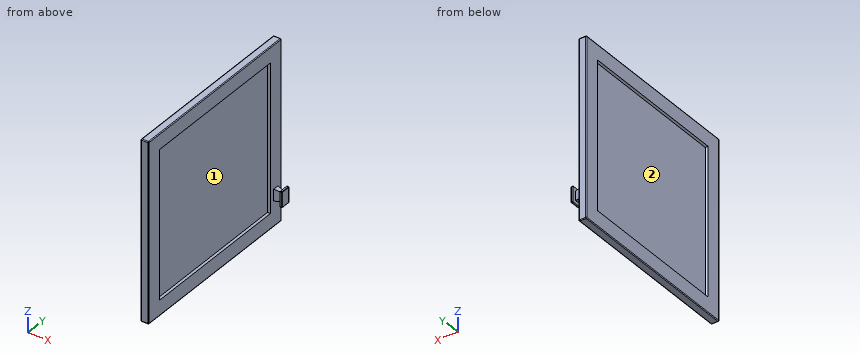
```python
from build123d import *

# Parameters (mm, degrees)
SKETCH1_W               = 479
SKETCH1_H               = 460
BOSS_EXTRUDE1_DEPTH     = 10
SKETCH2_W               = 399
SKETCH2_H               = 380
CUT_EXTRUDE1_DEPTH      = 5
CUT_EXTRUDE1_DRAFT      = -30
MIRROR1_COPY_1_SKETCH_W = 399
MIRROR1_COPY_1_SKETCH_H = 380
MIRROR1_COPY_1_DEPTH    = 5
MIRROR1_COPY_1_DRAFT    = -30
SKETCH3_W               = 15
SKETCH3_H               = 30
BOSS_EXTRUDE2_DEPTH     = 20
BOSS_EXTRUDE2_TAPER     = 10
SKETCH4_W               = 25
SKETCH4_H               = 40
BOSS_EXTRUDE3_DEPTH     = 5
FILLET3_R               = 2
FILLET4_R               = 1


with BuildPart() as part:
    # Sketch1 → Boss-Extrude1 (new, symmetric)
    with BuildSketch(Plane.YZ):
        with Locations((239.5, 230)):
            Rectangle(SKETCH1_W, SKETCH1_H)
    extrude(amount=BOSS_EXTRUDE1_DEPTH, both=True)


with BuildPart() as cut_extrude1_tool:
    # Sketch2 → Cut-Extrude1 (with draft: the straight prism first)
    with BuildSketch(Plane.YZ.offset(10)):
        with Locations((239.5, 230)):
            Rectangle(SKETCH2_W, SKETCH2_H)
    extrude(amount=-CUT_EXTRUDE1_DEPTH)
    # Cut-Extrude1: the draft: its side faces are tilted about the plane it starts from
    cut_extrude1_sides = [cut_extrude1_tool.faces().sort_by_distance(p)[0] for p in [
        (7.5, 40, 230),
        (7.5, 239.5, 40),
        (7.5, 439, 230),
        (7.5, 239.5, 420),
    ]]
    draft(cut_extrude1_sides, Plane.YZ.offset(10), CUT_EXTRUDE1_DRAFT)


with BuildPart() as part_1:
    add(part.part)

    # Cut-Extrude1: cut by cut_extrude1_tool
    add(cut_extrude1_tool.part, mode=Mode.SUBTRACT)


with BuildPart() as mirror1_copy_1_tool:
    # Mirror1 copy 1 sketch → Mirror1 copy 1 (with draft: the straight prism first)
    with BuildSketch(Plane(origin=(-10, 0, 0), x_dir=(0, 1, 0), z_dir=(-1, 0, 0))):
        with Locations((239.5, -230)):
            Rectangle(MIRROR1_COPY_1_SKETCH_W, MIRROR1_COPY_1_SKETCH_H)
    extrude(amount=-MIRROR1_COPY_1_DEPTH)
    # Mirror1 copy 1: the draft: its side faces are tilted about the plane it starts from
    mirror1_copy_1_sides = [mirror1_copy_1_tool.faces().sort_by_distance(p)[0] for p in [
        (-7.5, 40, 230),
        (-7.5, 239.5, 40),
        (-7.5, 439, 230),
        (-7.5, 239.5, 420),
    ]]
    draft(mirror1_copy_1_sides, Plane(origin=(-10, 0, 0), x_dir=(0, 1, 0), z_dir=(-1, 0, 0)), MIRROR1_COPY_1_DRAFT)


with BuildPart() as part_2:
    add(part_1.part)

    # Mirror1 copy 1: cut by mirror1_copy_1_tool
    add(mirror1_copy_1_tool.part, mode=Mode.SUBTRACT)

    # Sketch3 → Boss-Extrude2 (add)
    with BuildSketch(Plane.YZ.offset(10)):
        with Locations((459, 80)):
            Rectangle(SKETCH3_W, SKETCH3_H)
    extrude(amount=BOSS_EXTRUDE2_DEPTH, taper=BOSS_EXTRUDE2_TAPER)

    # Sketch4 → Boss-Extrude3 (add)
    with BuildSketch(Plane.YZ.offset(30)):
        with Locations((459, 80)):
            Rectangle(SKETCH4_W, SKETCH4_H)
    extrude(amount=BOSS_EXTRUDE3_DEPTH)

    # Fillet3
    fillet3_edges = [part_2.edges().sort_by_distance(p)[0] for p in [
        (10, 479, 230),
        (10, 239.5, 460),
        (10, 0, 230),
        (-10, 239.5, 460),
        (-10, 479, 230),
        (-10, 239.5, 0),
        (-10, 0, 230),
        (0, 0, 460),
        (0, 479, 460),
        (0, 479, 0),
        (0, 0, 0),
        (10, 239.5, 0),
    ]]
    fillet(fillet3_edges, radius=FILLET3_R)

    # Fillet4
    fillet4_edges = [part_2.edges().sort_by_distance(p)[0] for p in [
        (32.5, 446.5, 100),
        (32.5, 446.5, 60),
        (32.5, 471.5, 60),
        (32.5, 471.5, 100),
        (35, 446.5, 80),
        (35, 459, 60),
        (35, 471.5, 80),
        (35, 459, 100),
    ]]
    fillet(fillet4_edges, radius=FILLET4_R)


solid = part_2.part
```
Design review of the part built by this model. Coordinates are the model's own, in mm. Face numbers are marked on the shaded views. A direction names the side the tool comes from. Coordinates: 2 decimals unless noted, no trailing zeros. Order: outer loops, then holes, each group sorted by start corner. A loop starts at its lowest first (then second) coordinate and runs counter-clockwise, first axis right, second up. Notation, with made-up numbers: (-34.5, 76.25) - (-19.5, 76.25) arc R20 cw to (-19.5, 102.25) - close; hole circle Ø2 at (44.5, 20.25). An arc over 180 degrees is marked (long way). One line per question, with ' | ' between items.
Q1. Consider section B-B, the plane z = 256.5. Give the boundary of the cut face in (x, y).
Answer key:
outline: (-10, 2) arc R2 ccw to (-8, 0) - (8, 0) arc R2 ccw to (10, 2) - (10, 40) - (5, 42.89) - (5, 436.11) - (10, 439) - (10, 477) arc R2 ccw to (8, 479) - (-8, 479) arc R2 ccw to (-10, 477) - (-10, 439) - (-5, 436.11) - (-5, 42.89) - (-10, 40) - close
Q2. To check wall thickness, follow line 1 along X through (y, z) = (145, 64.5); line 2 along Y through (x, z) = (6, 137); line 3 along X through (y, z) = (340.5, 432). State the ranges of each line that lie inside material, in increasing order.
Answer key:
line 1: x = -5 to 5 | line 2: y = 0 to 42.31, 436.69 to 479 | line 3: x = -10 to 10
Q3. For the marked faces 1 and 2, list the 3-axis set-ups (+Z, -Z, +X, -X, +Y, -Y) from which the entire face can be reached by the end or side of a thin tool; tool diameter is ignored.
Answer key:
face 1: +X | face 2: -X
Q4. Consider section A-A, the plane y = 248.5. Give the boundary of the cut face in (x, z), then the cut area to 3 significant figures.
Answer key:
outline: (-10, 2) arc R2 ccw to (-8, 0) - (8, 0) arc R2 ccw to (10, 2) - (10, 40) - (5, 42.89) - (5, 417.11) - (10, 420) - (10, 458) arc R2 ccw to (8, 460) - (-8, 460) arc R2 ccw to (-10, 458) - (-10, 420) - (-5, 417.11) - (-5, 42.89) - (-10, 40) - close | area: 5,430 mm2
Q5. Clearance check with flat-ended pins moving along their axes: pin 1 Ø4.5 at (x, z) = (32, 89) entering from -Y; pin 2 Ø4.5 at (x, y) = (32, 461) entering from +Z; pin 3 Ø4 at (y, z) = (55, 96) entering from +X. State where each tip first meets the part, or that it passes through.
Answer key:
pin 1: stops at y = 446.5 | pin 2: stops at z = 100 | pin 3: stops at x = 5
